Work out the finished part from the listing and answer in its coordinate system (mm). Coordinates: 2 decimals unless noted, no trailing zeros. Order: outer loops, then holes, each group sorted by start corner. A loop starts at its lowest first (then second) coordinate and runs counter-clockwise, first axis right, second up. Notation, with made-up numbers: M 19,-3 L 33,-3 A36 ccw 33,35 Z; hole C 29,60.25 d11. An arc over 180 degrees is marked long. Use a Markdown table: item, result.
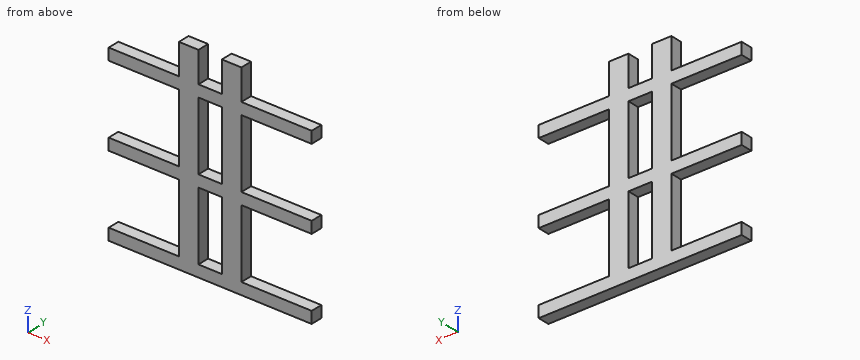
Autodesk Inventor part; units mm, degrees
ref_plane "YZ Plane" through (0, 0, 0) normal (1, 0, 0) x (0, 1, 0)
ref_plane "XZ Plane" through (0, 0, 0) normal (0, 1, 0) x (-1, 0, 0)
ref_plane "XY Plane" through (0, 0, 0) normal (0, 0, 1) x (1, 0, 0)
sketch "Sketch1" plane through (0, 0, 0) normal (0, 1, 0) x (-1, 0, 0)
  line L0 (0, 0) -> (-5, 0)
  line L1 (-5, 0) -> (-5, 50)
  line L2 (-5, 50) -> (0, 50)
  line L3 (0, 50) -> (0, 0)
  line L4 (-16, 50) -> (-11, 50)
  line L5 (-11, 50) -> (-11, 0)
  line L6 (-11, 0) -> (-16, 0)
  line L7 (-16, 0) -> (-16, 50)
  line L8 (18, 1) -> (-34, 1)
  line L9 (-34, 1) -> (-34, -2)
  line L10 (-34, -2) -> (18, -2)
  line L11 (18, -2) -> (18, 1)
  line L12 (-5, 0) -> (-11, 0)
  line L13 (18, 18.56) -> (-34, 18.56)
  line L14 (-34, 18.56) -> (-34, 21.56)
  line L15 (-34, 21.56) -> (18, 21.56)
  line L16 (18, 21.56) -> (18, 18.56)
  line L17 (18, 39.12) -> (-34, 39.12)
  line L18 (-34, 39.12) -> (-34, 42.12)
  line L19 (-34, 42.12) -> (18, 42.12)
  line L20 (18, 42.12) -> (18, 39.12)
  point P0 (-8, 0)
  point P1 (-8, -2)
  point P2 (0, 18.56)
  point P3 (0, 21.56)
  point P4 (0, 39.12)
  point P5 (0, 42.12)
  point P6 (-5, 42.12)
  point P7 (-11, 42.12)
  point P8 (-16, 42.12)
  point P9 (-16, 39.12)
  point P10 (-16, 21.56)
  point P11 (-16, 18.56)
  point P12 (-16, 1)
  point P13 (0, 1)
  point P14 (-11, 21.56)
  point P15 (-11, 39.12)
  point P16 (-5, 39.12)
  point P17 (-5, 21.56)
  point P18 (-5, 18.56)
  point P19 (-5, 1)
  point P20 (-11, 1)
  point P21 (-11, 18.56)
  point P22 (-8, 18.56)
  dimension "d0" = 5
  dimension "d1" = 50
  dimension "d3" = 5
  dimension "d4" = 50
  dimension "d5" = 52
  dimension "d6" = 3
  dimension "d7" = 1
  dimension "d8" = 0
  dimension "d9" = 52
  dimension "d10" = 3
  dimension "d11" = 52
  dimension "d12" = 3
  dimension "d16" = 20.56
  dimension "d17" = 20.56
  dimension "d20" = 16
  dimension "d21" = 0
extrude "Extrusion1" add sketch "Sketch1" along normal blind 3 contours L3 L8 L11 L10 L9 L7 L6 L12 L0 | L0 L1 L8 L3 | L12 L5 L8 L1 | L8 L1 L13 L3 | L6 L7 L8 L5 | L13 L1 L15 L3 | L3 L15 L16 L13 | L13 L5 L15 L1 | L8 L7 L13 L5 | L15 L1 L17 L3 | L13 L7 L15 L5 | L17 L1 L19 L3 | L3 L19 L20 L17 | L17 L5 L19 L1 | L15 L7 L17 L5 | L13 L14 L15 L7 | L19 L1 L2 L3 | L17 L7 L19 L5 | L19 L7 L4 L5 | L17 L18 L19 L7
equation "\"d3\" = d0"
equation "\"d4\" = d1"
properties part number "module-switch_port-catch" material "PC/ABS Plastic"
1. Find the intervals of material crossed by probe 1 along Z at (x, y) = (-14.5, 2.2); probe 2 along X at (y, z) = (1.6, 18.5), in increasing order.
Answers below:
| item | result |
|---|---|
| probe 1 | -2 to 1, 18.56 to 21.56, 39.12 to 42.12 |
| probe 2 | 0 to 5, 11 to 16 |
2. Section B-B on x = 6 is taken. Determine the outline of the cut face in (y, z).
Answers below:
| item | result |
|---|---|
| outline | M 0,-2 L 3,-2 L 3,1 L 0,1 Z; M 0,18.56 L 3,18.56 L 3,21.56 L 0,21.56 Z; M 0,39.12 L 3,39.12 L 3,42.12 L 0,42.12 Z |
3. Section A-A on z = 33.5 is taken. Determine the outline of the cut face in (x, y), then the cut area to 3 significant figures.
Answers below:
| item | result |
|---|---|
| outline | M 0,0 L 5,0 L 5,3 L 0,3 Z; M 11,0 L 16,0 L 16,3 L 11,3 Z |
| area | 30.0 mm² |
4. Section C-C on y = 1.45 is taken. Give the number of separate pieces and of enclosed holes in the cut face, then the cut area to 3 significant figures.
Answers below:
| item | result |
|---|---|
| separate pieces | 1 |
| enclosed holes | 2 |
| area | 898 mm² |
5. Flat-ended cylindrical pins translate along their axes: P1, Ø1.5, axis at y = 2, z = 27, coming from the +X side; P2, Ø1, axis at x = 11, z = 42, coming from the -Y side. Find the tip coordinate at first contact, or state that the pin passes through.
Answers below:
| item | result |
|---|---|
| P1 | x = 16 |
| P2 | y = 0 |
